Here's how the part is built. I have some questions about the finished solid (model axes, mm). Coordinates: 2 decimals unless noted, no trailing zeros. Write each loop counter-clockwise with the first axis right and the second up, starting at its lowest first coordinate (ties: lowest second). Pieces come first, ordered by that corner, then holes.
(1) Imagine slicing it at D-D, the plane x = 19. List the corners of the cut face in (y, z) for me, plus the area to 3 significant figures.
(2) Imagine slicing it at B-B, the plane x = 0. List the corners of the cut face in (y, z) for me.
(3) Imagine slicing it at C-C, the plane z = -35.5. List the corners of the cut face in (x, y) for me.
(4) Please list where these lines run through material, in increasing order: probe 1 along Z at (x, y) = (0, 0.25); probe 2 along X at (y, z) = (-10.5, 35.5); probe 3 along X at (y, z) = (-7, -39).
(5) Thinking about a two-plate mould opening in Z: for faces 1 (the cylindrical face through (-8.71, -0.18, -6.9)), 2 (the flat face through (-7, -12.7, 0)), which applies, released by +Z, released by -Z, zero draft, split by the parting line, or undercut?
(6) Imagine slicing it at A-A, the plane y = 8.25. State how many separate pieces and enclosed holes the cut face has, plus the area to 3 significant figures.
(7) For pin 1 Ø2 at (x, y) = (-24.5, -5) entering from -Z; pin 2 Ø3 at (x, y) = (27.5, -5.5) entering from +Z; pin 3 Ø4 at (y, z) = (4.5, -10) entering from -X, each with a flat end and sliding along its axis, tell me the tip position at first contact or that it passes through.
Autodesk Inventor part; units mm, degrees
ref_plane "YZ Plane" through (0, 0, 0) normal (1, 0, 0) x (0, 1, 0)
ref_plane "XZ Plane" through (0, 0, 0) normal (0, 1, 0) x (-1, 0, 0)
ref_plane "XY Plane" through (0, 0, 0) normal (0, 0, 1) x (1, 0, 0)
sketch "Sketch1" plane through (0, 0, 0) normal (0, 1, 0) x (-1, 0, 0)
  circle A0 centre (0, 0) radius 6.35
  circle A1 centre (0, 0) radius 50.8
  arc A2 (-17.8028, -42.456) -> (17.8028, -42.456) centre (0, 0) ccw
  line L0 (0, 0) -> (0, -50.8) construction
  arc A3 (-2.5641, -10.8126) -> (2.5641, -10.8126) centre (0, 0) ccw
  line L1 (17.8028, -42.456) -> (2.5641, -10.8126)
  line L2 (-2.5641, -10.8126) -> (-17.8028, -42.456)
  line L3 (6.855, -8.7463) -> (22.0936, -40.3896)
  arc A4 (22.0936, -40.3896) -> (44.2933, -12.5521) centre (0, 0) ccw
  line L4 (44.2933, -12.5521) -> (10.0523, -4.7369)
  arc A5 (6.855, -8.7463) -> (10.0523, -4.7369) centre (0, 0) ccw
  line L5 (11.1121, -0.0938) -> (45.353, -7.909)
  arc A6 (45.353, -7.909) -> (37.4301, 26.8038) centre (0, 0) ccw
  line L6 (37.4301, 26.8038) -> (9.971, 4.9059)
  arc A7 (11.1121, -0.0938) -> (9.971, 4.9059) centre (0, 0) ccw
  line L7 (7.0016, 8.6293) -> (34.4607, 30.5272)
  arc A8 (34.4607, 30.5272) -> (2.3812, 45.9759) centre (0, 0) ccw
  line L8 (2.3812, 45.9759) -> (2.3812, 10.8544)
  arc A9 (7.0016, 8.6293) -> (2.3812, 10.8544) centre (0, 0) ccw
  line L9 (-2.3813, 10.8544) -> (-2.3813, 45.9759)
  arc A10 (-2.3813, 45.9759) -> (-34.4607, 30.5272) centre (0, 0) ccw
  line L10 (-34.4607, 30.5272) -> (-7.0016, 8.6293)
  arc A11 (-2.3813, 10.8544) -> (-7.0016, 8.6293) centre (0, 0) ccw
  line L11 (-9.971, 4.9059) -> (-37.4301, 26.8038)
  arc A12 (-37.4301, 26.8038) -> (-45.353, -7.909) centre (0, 0) ccw
  line L12 (-45.353, -7.909) -> (-11.1121, -0.0938)
  arc A13 (-9.971, 4.9059) -> (-11.1121, -0.0938) centre (0, 0) ccw
  line L13 (-10.0523, -4.7369) -> (-44.2933, -12.5521)
  arc A14 (-44.2933, -12.5521) -> (-22.0936, -40.3896) centre (0, 0) ccw
  line L14 (-22.0936, -40.3896) -> (-6.855, -8.7463)
  arc A15 (-10.0523, -4.7369) -> (-6.855, -8.7463) centre (0, 0) ccw
  point P0 (0, -46.0375)
  point P1 (0, -11.1125)
  point P2 (35.9936, -28.7039)
  point P3 (8.6881, -6.9285)
  point P4 (44.8832, 10.2443)
  point P5 (10.8339, 2.4728)
  point P6 (19.9749, 41.4784)
  point P7 (4.8215, 10.012)
  point P8 (-19.9749, 41.4784)
  point P9 (-4.8215, 10.012)
  point P10 (-44.8832, 10.2443)
  point P11 (-10.8339, 2.4728)
  point P12 (-35.9936, -28.7039)
  point P13 (-8.6881, -6.9285)
  dimension "d1" = 101.6
  dimension "d0" = 12.7
  dimension "d4" = 4.7625
  dimension "d5" = 4.7625
  dimension "d8" = 360
  dimension "d10" = 4.7625
extrude "Extrusion1" add sketch "Sketch1" along normal mid plane 25.4
equation "\"d5\" = d4"
equation "\"d10\" = d4"
properties part number "intake roller" material "Rubber"
Recorded:
1. outline: (-12.7, -47.11) - (12.7, -47.11) - (12.7, -33.97) - (-12.7, -33.97) - close; (-12.7, -6.78) - (12.7, -6.78) - (12.7, -1.89) - (-12.7, -1.89) - close; (-12.7, 12.11) - (12.7, 12.11) - (12.7, 18.2) - (-12.7, 18.2) - close; (-12.7, 41.93) - (12.7, 41.93) - (12.7, 47.11) - (-12.7, 47.11) - close
1. area: 744 mm2
2. outline: (-12.7, -50.8) - (12.7, -50.8) - (12.7, -46.04) - (-12.7, -46.04) - close; (-12.7, -11.11) - (12.7, -11.11) - (12.7, -6.35) - (-12.7, -6.35) - close; (-12.7, 6.35) - (12.7, 6.35) - (12.7, 50.8) - (-12.7, 50.8) - close
3. outline: (-36.34, -12.7) - (-29.31, -12.7) - (-29.31, 12.7) - (-36.34, 12.7) - close; (-19.74, -12.7) - (-14.45, -12.7) - (-14.45, 12.7) - (-19.74, 12.7) - close; (14.45, -12.7) - (19.74, -12.7) - (19.74, 12.7) - (14.45, 12.7) - close; (29.31, -12.7) - (36.34, -12.7) - (36.34, 12.7) - (29.31, 12.7) - close
4. probe 1: z = -50.8 to -46.04, -11.11 to -6.35, 6.35 to 50.8
4. probe 2: x = -36.34 to -29.31, -2.38 to 2.38, 29.31 to 36.34
4. probe 3: x = -32.55 to -24.46, -21.42 to -16.14, 16.14 to 21.42, 24.46 to 32.55
5. face 1: undercut
5. face 2: zero draft
6. separate pieces: 1
6. enclosed holes: 8
6. area: 2,880 mm2
7. pin 1: stops at z = -45.04
7. pin 2: stops at z = 43.64
7. pin 3: stops at x = -50.17
